For this review, use the dimensioned drawing (mm, ordinates from the lowest corner) and the shaded views. A direction names the side the tool comes from. Give positions to 0.01 mm unless a question says otherwise; leave off trailing zeros. Loops run counter-clockwise (first coordinate to the right, second up) from the corner with the lowest first, then second, coordinate; pieces in that order, holes last. Notation, with made-up numbers: M 33,49.5 L 41,49.5 A23 cw 41,84.5 Z; hole C 34,-14 d1. An arc over 180 degrees is marked long. Use CSV: the item, a comma, the result in double quotes. Start each with the question number.
1. Take a section at C-C, the plane z = 679.5. Write out the cut boundary in (x, y).
2. Take a section at B-B, the plane y = 42. Write out the cut boundary in (x, z), and give its area (3 significant figures).
3. Take a section at A-A, the plane z = 119. Write out the cut boundary in (x, y).
4. To check wall thickness, follow line 1 (Y direction, x = 3, z = 119); line 2 (Y direction, x = 5.5, z = 721); line 3 (Y direction, x = 58, z = 332). State the ranges of each line that lie inside material, in increasing order. Write a range as [from, to].
5. Tool access review of the marked faces 1 and 2: name each direction out of +Z, -Z, +X, -X, +Y, -Y from which nothing blocks a thin tool from reaching the whole face with its end or side.
6. Take a section at D-D, the plane x = 72. Write out the cut boundary in (y, z), and give its area (3 significant figures).
7. Insertion check: P1, Ø4, axis at y = 6, z = 34.5, coming from the +X side. The pin has a flat end and moves straight along its axis. Give the tip position at first contact, or say it passes through.
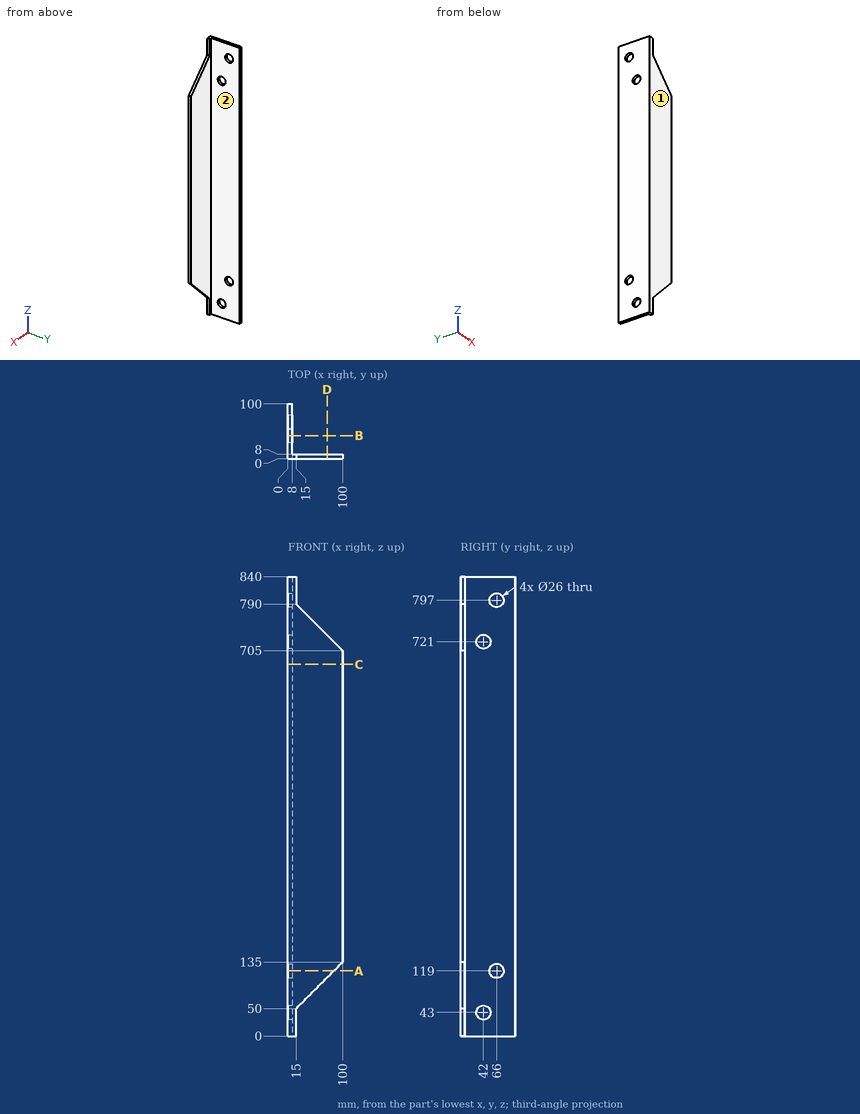
Result set:
1,outline,"M 0,0 L 100,0 L 100,8 L 8,8 L 8,100 L 0,100 Z"
2,outline,"M 0,0 L 8,0 L 8,30 L 0,30 Z; M 0,56 L 8,56 L 8,708 L 0,708 Z; M 0,734 L 8,734 L 8,840 L 0,840 Z"
2,area,"6,300 mm2"
3,outline,"M 0,0 L 84,0 L 84,8 L 8,8 L 8,53 L 0,53 Z; M 0,79 L 8,79 L 8,100 L 0,100 Z"
4,line 1,"[0, 53], [79, 100]"
4,line 2,"[0, 29], [55, 100]"
4,line 3,"[0, 8]"
5,face 1,"+Z, -Z, +X, -X, -Y"
5,face 2,"+Z, -Z, +X, +Y"
6,outline,"M 0,107 L 8,107 L 8,733 L 0,733 Z"
6,area,"5,010 mm2"
7,P1,"x = 15"
